```python
from build123d import *

# Parameters (mm, degrees)
SKETCH_1_R               = 17.5
SKETCH_1_R_2             = 15.25
SKETCH_1_R_3             = 14.1
EXTRUDE_1_DEPTH          = 2.5
SKETCH_1_3_R             = 15.25
SKETCH_1_3_R_2           = 14.1
EXTRUDE_2_DEPTH          = 14
CUT_EXTRUDE_START        = 5.5
SKETCH_1_4_R             = 15.25
SKETCH_1_4_R_2           = 14.1
CUT_EXTRUDE_1_DEPTH      = 2.6
CUT_EXTRUDE_START_2      = 9.5
SKETCH_1_5_R             = 15.25
SKETCH_1_5_R_2           = 14.1
CUT_EXTRUDE_2_DEPTH      = 2.6
CHAMFER_1_SIZE           = 0.5
SKETCH_2_R               = 5
CUT_EXTRUDE_5_DEPTH      = 30.744747435
CUT_EXTRUDE_START_3      = 10
SKETCH_4_R               = 1.25
CUT_EXTRUDE_6_DEPTH      = 19.434134416
PATTERN_CIRCULAR_1_COUNT = 4


with BuildPart() as part:
    # Sketch 1 → Extrude 1 (new body)
    # profile 1 of 3: a face of its own
    with BuildSketch(Plane.XY):
        Circle(SKETCH_1_R)
        Circle(SKETCH_1_R_2, mode=Mode.SUBTRACT)
    # profile 2 of 3: a face of its own
    with BuildSketch(Plane.XY):
        Circle(SKETCH_1_R_2)
        Circle(SKETCH_1_R_3, mode=Mode.SUBTRACT)
    # profile 3 of 3: a face of its own
    with BuildSketch(Plane.XY):
        Circle(SKETCH_1_R_3)
    extrude(amount=-EXTRUDE_1_DEPTH)

    # Sketch 1_3 → Extrude 2 (add)
    # profile 1 of 2: a face of its own
    with BuildSketch(Plane.XY):
        Circle(SKETCH_1_3_R)
        Circle(SKETCH_1_3_R_2, mode=Mode.SUBTRACT)
    # profile 2 of 2: a face of its own
    with BuildSketch(Plane.XY):
        Circle(SKETCH_1_3_R_2)
    extrude(amount=EXTRUDE_2_DEPTH)

    # Sketch 1_4 → Cut-Extrude 1 (cut)
    with BuildSketch(Plane.XY.offset(CUT_EXTRUDE_START)):
        Circle(SKETCH_1_4_R)
        Circle(SKETCH_1_4_R_2, mode=Mode.SUBTRACT)
    extrude(amount=CUT_EXTRUDE_1_DEPTH, mode=Mode.SUBTRACT)

    # Sketch 1_5 → Cut-Extrude 2 (cut)
    with BuildSketch(Plane.XY.offset(CUT_EXTRUDE_START_2)):
        Circle(SKETCH_1_5_R)
        Circle(SKETCH_1_5_R_2, mode=Mode.SUBTRACT)
    extrude(amount=CUT_EXTRUDE_2_DEPTH, mode=Mode.SUBTRACT)

    # Chamfer 1
    chamfer_1_edges = [part.edges().sort_by_distance(p)[0] for p in [
        (-17.5, 0, 0),
        (-17.5, 0, -2.5),
        (-15.25, 0, 14),
    ]]
    chamfer(chamfer_1_edges, length=CHAMFER_1_SIZE)

    # Sketch 2 → Cut-Extrude 5 (cut, through all)
    with BuildSketch(Plane(origin=(0, 0, -2.5), x_dir=(-1, 0, 0), z_dir=(0, 0, -1))):
        with Locations((-6, 0)):
            Circle(SKETCH_2_R)
    extrude(amount=-CUT_EXTRUDE_5_DEPTH, mode=Mode.SUBTRACT)

    # Sketch 4 → Cut-Extrude 6 (cut, through all)
    with BuildSketch(Plane(origin=(0, 0, 0), x_dir=(0, 0, -1), z_dir=(0.7071067811865488, 0.7071067811865464, 0)).offset(CUT_EXTRUDE_START_3)):
        with Locations(Location((-3, 0, 0), (0, 0, 270))):
            Circle(SKETCH_4_R)
    cut_extrude_6 = extrude(amount=CUT_EXTRUDE_6_DEPTH, mode=Mode.SUBTRACT)

    # Pattern Circular 1: Cut-Extrude 6 ×4 about axis
    pattern_circular_1_axis = Axis((0, 0, 0), (0, 0, 1))
    for i in range(1, PATTERN_CIRCULAR_1_COUNT):
        add(cut_extrude_6.rotate(pattern_circular_1_axis, i * 360 / PATTERN_CIRCULAR_1_COUNT), mode=Mode.SUBTRACT)


solid = part.part
```
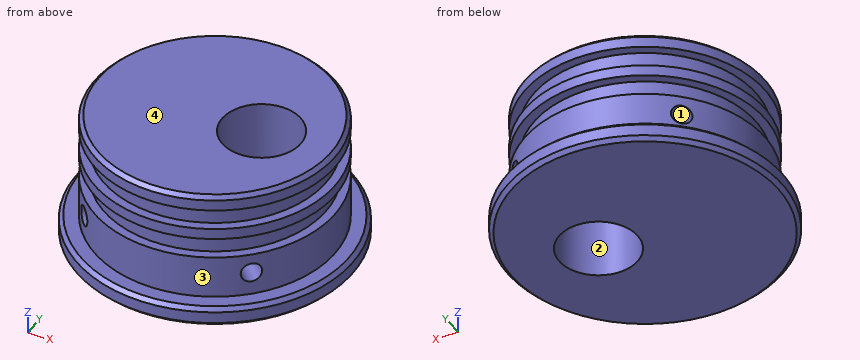
For this review, take the finished solid that the model builds, in its own axes (mm). Face numbers are marked on the shaded views. Round coordinates to 2 decimals unless told otherwise and drop trailing zeros. Write each loop counter-clockwise with the first axis right and the second up, starting at its lowest first coordinate (ties: lowest second). Pieces come first, ordered by that corner, then holes. Notation, with made-up numbers: (70, 24) -> (123, 24) arc R23 cw to (123, 46) -> close; hole circle Ø8 at (-40, -6). An arc over 180 degrees is marked (long way). Use one line per item in the form item = value.
1) Clearance check with flat-ended pins moving along their axes: pin 1 (2 mm diameter, centred on x = -6.5, z = 5.5, fed in from +Y); pin 2 (3 mm diameter, centred on y = 11, z = 11.5, fed in from -X); pin 3 (4 mm diameter, centred on y = 9, z = 3, fed in from +X); pin 4 (8 mm diameter, centred on x = 6, y = 0, fed in from +Z). State where each tip first meets the part, or that it passes through.
Found:
pin_1 = 14.22
pin_2 = -11.83
pin_3 = 13.55
pin_4 = through
2) Mouldability with a two-part tool opening along Y and no side actions: class the marked faces 1, 2, 3 and 4 as +Y half, -Y half, draft (parallel to the pull), parting line (faces both ways), or undercut.
Found:
face_1 = undercut
face_2 = undercut
face_3 = parting line
face_4 = draft
3) To check wall thickness, follow L1, parallel to Z at x = -11.5, y = 9; L2, parallel to X at y = -9.5, z = 3.5; L3, parallel to X at y = 2, z = 12. State the ranges of each line that lie inside material, in increasing order. Write a range as from..to.
Found:
L1 = -2.5..5.5, 8.1..9.5, 12.1..14
L2 = -11.93..-11.12, -7.88..7.88, 11.12..11.93
L3 = -13.96..1.42, 10.58..13.96
4) Take a section at D-D, the plane x = -7.5. Count the separate pieces of the cut face and the enclosed holes in it, and give its area (3 significant figures).
Found:
separate_pieces = 1
enclosed_holes = 2
area = 425 mm2
5) Take a section at C-C, the plane z = 3.5. Write out the cut boundary in (x, y).
Found:
outline = (-11.56, -9.94) -> (-7.88, -6.26) -> (-6.26, -7.88) -> (-9.94, -11.56) arc R15.25 ccw to (9.94, -11.56) -> (6.26, -7.88) -> (7.88, -6.26) -> (11.56, -9.94) arc R15.25 ccw to (11.56, 9.94) -> (7.88, 6.26) -> (6.26, 7.88) -> (9.94, 11.56) arc R15.25 ccw to (-9.94, 11.56) -> (-6.26, 7.88) -> (-7.88, 6.26) -> (-11.56, 9.94) arc R15.25 ccw to start; hole circle Ø10 at (6, 0)
